The listing builds one solid part. Answer for the finished solid, in the listing's coordinates (mm). A direction names the side the tool comes from. Round coordinates to 2 decimals unless told otherwise and drop trailing zeros. Write each loop counter-clockwise with the first axis right and the second up, starting at its lowest first coordinate (ties: lowest second). Pieces come first, ordered by that corner, then holes. Notation, with made-up numbers: (32, 6.5) - (42, 6.5) arc R25 ccw to (42, 45.5) - close; hole circle Ø9 at (45.25, -29.5). An arc over 180 degrees is marked (long way). Answer in a Markdown table with one row per item.
from build123d import *

# Parameters (mm, degrees)
BOSS_EXTRUDE1_DEPTH  = 100
BOSS_EXTRUDE2_DEPTH  = 10
BOSS_EXTRUDE2_DRAFT  = 45
SKETCH3_R            = 34.5
BOSS_EXTRUDE3_DEPTH  = 10
SKETCH4_R            = 31
BOSS_EXTRUDE4_DEPTH  = 30
SKETCH5_R            = 2.5
SKETCH5_R_2          = 2
BOSS_EXTRUDE5_DEPTH  = 1
CIRPATTERN1_COUNT    = 12
BOSS_EXTRUDE6_DEPTH  = 100
SKETCH7_R            = 31
BOSS_EXTRUDE7_DEPTH  = 10
SKETCH8_R            = 30
BOSS_EXTRUDE8_DEPTH  = 1
SKETCH9_R            = 31
BOSS_EXTRUDE9_DEPTH  = 10
SKETCH10_R           = 42.5
BOSS_EXTRUDE10_DEPTH = 10.5
BOSS_EXTRUDE11_DEPTH = 35
BOSS_EXTRUDE12_DEPTH = 40
CUT_EXTRUDE1_DEPTH   = 40
SKETCH14_R           = 15
CUT_EXTRUDE2_DEPTH   = 20
SKETCH15_R           = 15
CUT_EXTRUDE3_DEPTH   = 20


with BuildPart() as part:
    # Sketch1 → Boss-Extrude1 (new body)
    with BuildSketch(Plane(origin=(0, 0, 0), x_dir=(0, 0, -1), z_dir=(1, 0, 0))):
        with BuildLine():
            Line((-37.5, 45), (37.5, 45))
            ThreePointArc((37.5, 45), (45.880962103, 0), (37.5, -45))
            Line((37.5, -45), (-37.5, -45))
            ThreePointArc((-37.5, -45), (-45.880962103, 0), (-37.5, 45))
        make_face()
    extrude(amount=BOSS_EXTRUDE1_DEPTH)


with BuildPart() as boss_extrude2_tool:
    # Sketch2 → Boss-Extrude2 (with draft: the straight prism first)
    with BuildSketch(Plane(origin=(100, 0, 0), x_dir=(0, 0, -1), z_dir=(1, 0, 0))):
        with BuildLine():
            Line((37.5, 45), (-37.5, 45))
            ThreePointArc((-37.5, 45), (-45.880962103, 0), (-37.5, -45))
            Line((-37.5, -45), (37.5, -45))
            ThreePointArc((37.5, -45), (45.880962103, 0), (37.5, 45))
        make_face()
    extrude(amount=BOSS_EXTRUDE2_DEPTH)
    # Boss-Extrude2: the draft: its side faces are tilted about the plane it starts from
    boss_extrude2_sides = [boss_extrude2_tool.faces().sort_by_distance(p)[0] for p in [
        (105, -45, 0),
        (105, 0, -45.880962103),
        (105, 45, 0),
        (105, 0, 45.880962103),
    ]]
    draft(boss_extrude2_sides, Plane(origin=(100, 0, 0), x_dir=(0, 0, -1), z_dir=(1, 0, 0)), BOSS_EXTRUDE2_DRAFT)


with BuildPart() as part_1:
    add(part.part)

    # Boss-Extrude2: add boss_extrude2_tool
    add(boss_extrude2_tool.part)

    # Sketch3 → Boss-Extrude3 (add)
    with BuildSketch(Plane(origin=(110, 0, 0), x_dir=(0, 0, -1), z_dir=(1, 0, 0))):
        Circle(SKETCH3_R)
    extrude(amount=BOSS_EXTRUDE3_DEPTH)

    # Sketch4 → Boss-Extrude4 (add)
    with BuildSketch(Plane(origin=(120, 0, 0), x_dir=(0, 0, -1), z_dir=(1, 0, 0))):
        Circle(SKETCH4_R)
    extrude(amount=BOSS_EXTRUDE4_DEPTH)

    # Sketch5 → Boss-Extrude5 (add)
    with BuildSketch(Plane(origin=(150, 0, 0), x_dir=(0, 0, -1), z_dir=(1, 0, 0))):
        with Locations((27, 0)):
            Circle(SKETCH5_R)
        with Locations((27, 0)):
            Circle(SKETCH5_R_2, mode=Mode.SUBTRACT)
    boss_extrude5 = extrude(amount=BOSS_EXTRUDE5_DEPTH)

    # CirPattern1: Boss-Extrude5 ×12 about axis
    cirpattern1_axis = Axis((0, 0, 0.17674784), (1, 0, 0))
    for i in range(1, CIRPATTERN1_COUNT):
        add(boss_extrude5.rotate(cirpattern1_axis, i * 360 / CIRPATTERN1_COUNT))

    # Sketch6 → Boss-Extrude6 (add)
    with BuildSketch(Plane(origin=(150, 0, 0), x_dir=(0, 0, -1), z_dir=(1, 0, 0))):
        with BuildLine():
            Line((16, 0), (16, 17))
            ThreePointArc((16, 17), (0, 23.900331129), (-16, 17))
            Line((-16, 17), (-16, 0))
            Line((-16, 0), (-16, -17))
            ThreePointArc((-16, -17), (0, -23.900331129), (16, -17))
            Line((16, -17), (16, 0))
        make_face()
    extrude(amount=BOSS_EXTRUDE6_DEPTH)

    # Sketch7 → Boss-Extrude7 (add)
    with BuildSketch(Plane(origin=(250, 0, 0), x_dir=(0, 0, -1), z_dir=(1, 0, 0))):
        Circle(SKETCH7_R)
    extrude(amount=BOSS_EXTRUDE7_DEPTH)

    # Sketch8 → Boss-Extrude8 (add)
    with BuildSketch(Plane(origin=(260, 0, 0), x_dir=(0, 0, -1), z_dir=(1, 0, 0))):
        Circle(SKETCH8_R)
    extrude(amount=BOSS_EXTRUDE8_DEPTH)

    # Sketch9 → Boss-Extrude9 (add)
    with BuildSketch(Plane(origin=(261, 0, 0), x_dir=(0, 0, -1), z_dir=(1, 0, 0))):
        Circle(SKETCH9_R)
    extrude(amount=BOSS_EXTRUDE9_DEPTH)

    # Sketch10 → Boss-Extrude10 (add, symmetric)
    with BuildSketch(Plane.XY.offset(37.5)):
        with Locations((50, -45)):
            Circle(SKETCH10_R)
    extrude(amount=BOSS_EXTRUDE10_DEPTH, both=True)

    # Sketch11 → Boss-Extrude11 (add)
    with BuildSketch(Plane(origin=(0, 0, 27), x_dir=(-1, 0, 0), z_dir=(0, 0, -1))):
        with BuildLine():
            Line((-62.06556146, -45), (-22.06556146, -45))
            Line((-22.06556146, -45), (-22.06556146, -75))
            ThreePointArc((-22.06556146, -75), (-42.06556146, -82.639320225), (-62.06556146, -75))
            Line((-62.06556146, -75), (-62.06556146, -45))
        make_face()
    extrude(amount=BOSS_EXTRUDE11_DEPTH)

    # Sketch12 → Boss-Extrude12 (add)
    with BuildSketch(Plane(origin=(62.06556146, 0, 0), x_dir=(0, 0, -1), z_dir=(1, 0, 0))):
        with BuildLine():
            Line((8, -45), (33, -45))
            ThreePointArc((33, -45), (25.421855105, -68.929675658), (8, -87))
            Line((8, -87), (8, -45))
        make_face()
    extrude(amount=-BOSS_EXTRUDE12_DEPTH)

    # Sketch13 → Cut-Extrude1 (cut)
    with BuildSketch(Plane.XY.offset(-8)):
        with BuildLine():
            Line((22.06556146, -75), (22.06556146, -87))
            Line((22.06556146, -87), (62.06556146, -87))
            Line((62.06556146, -87), (62.06556146, -75))
            ThreePointArc((62.06556146, -75), (42.06556146, -82.639320225), (22.06556146, -75))
        make_face()
    extrude(amount=-CUT_EXTRUDE1_DEPTH, mode=Mode.SUBTRACT)

    # Sketch14 → Cut-Extrude2 (cut)
    with BuildSketch(Plane(origin=(271, 0, 0), x_dir=(0, 0, -1), z_dir=(1, 0, 0))):
        Circle(SKETCH14_R)
    extrude(amount=-CUT_EXTRUDE2_DEPTH, mode=Mode.SUBTRACT)

    # Sketch15 → Cut-Extrude3 (cut)
    with BuildSketch(Plane.XY.offset(48)):
        with Locations((50, -45)):
            Circle(SKETCH15_R)
    extrude(amount=-CUT_EXTRUDE3_DEPTH, mode=Mode.SUBTRACT)


solid = part_1.part
(1) For faces 1 (the flat face through (68, -61, 27)), 2 (the flat face through (151, -12, 22)), 3 (the flat face through (251, 0, 0)), 4 (the flat face through (50, -45, 28)), 5 (the cylindrical face through (150.493, -21.095, -13.954)), determine the directions among +Z, -Z, +X, -X, +Y, -Y from which every point of the face is accessible in a straight line to the end or side of a thin tool.
Checked values:
| item | result |
|---|---|
| face 1 | -Z, -Y |
| face 2 | +Z, +Y, -Y |
| face 3 | +X |
| face 4 | +Z |
| face 5 | none |
(2) For a pull along X with two mould halves and no side action, classify faces 6 (the cylindrical face through (254.93, 30.736, 4.036)), 7 (the flat face through (62.066, -60, -3)), 8 (the cylindrical face through (150.49, -13.91, 26.19)) as pulls with the +X half, pulls with the -X half, needs draft (parallel to the pull), parting line crosses it, or undercut.
Checked values:
| item | result |
|---|---|
| face 6 | needs draft |
| face 7 | pulls with the +X half |
| face 8 | undercut |
(3) Flat-ended cylindrical pins translate along their axes: pin 1 (3 mm diameter, centred on x = 195, y = -18, fed in from -Z); pin 2 (12 mm diameter, centred on x = 43.5, y = -73.5, fed in from -Z); pin 3 (4 mm diameter, centred on x = 125.5, y = -23, fed in from +Z). Find the tip coordinate at first contact, or state that the pin passes through.
Checked values:
| item | result |
|---|---|
| pin 1 | stops at z = -16 |
| pin 2 | stops at z = -26.24 |
| pin 3 | stops at z = 22.8 |
(4) Section A-A (x = 45.5) is taken. Give the vertices of the cut face in (y, z).
Checked values:
| item | result |
|---|---|
| outline | (-87.26, 27) - (-82.44, 27) - (-82.44, -14.09) arc R55 ccw to (-45, -33) - (-45, -37.5) arc R125 ccw to (45, -37.5) - (45, 37.5) arc R125 ccw to (-2.74, 45.85) - (-2.74, 48) - (-30.69, 48) - (-30.69, 28) - (-59.31, 28) - (-59.31, 48) - (-87.26, 48) - close |
(5) Section B-B (y = -50.5) is taken. Give the vertices of the cut face in (x, z), and give its area (3 significant figures).
Checked values:
| item | result |
|---|---|
| outline | (7.86, 27) - (22.07, 27) - (22.07, -32.3) - (62.07, -32.3) - (62.07, 27) - (92.14, 27) - (92.14, 48) - (63.96, 48) - (63.96, 28) - (36.04, 28) - (36.04, 48) - (7.86, 48) - close |
| area | 3,580 mm2 |
(6) Section C-C (x = 209.5) is taken. Give the vertices of the cut face in (y, z).
Checked values:
| item | result |
|---|---|
| outline | (-17, -16) - (17, -16) arc R22 ccw to (17, 16) - (-17, 16) arc R22 ccw to start |
(7) Find the intervals of material crossed by line 1 (X direction, y = -17.5, z = -20.5); line 2 (X direction, y = 24, z = -29); line 3 (Y direction, x = 19, z = 16.5), in increasing order.
Checked values:
| item | result |
|---|---|
| line 1 | x = 0 to 150, 250 to 271 |
| line 2 | x = 0 to 110 |
| line 3 | y = -45 to 45 |
(8) Section D-D (y = -65) is taken. Give the vertices of the cut face in (x, z).
Checked values:
| item | result |
|---|---|
| outline | (12.5, 27) - (22.07, 27) - (22.07, -27.55) - (62.07, -27.55) - (62.07, 27) - (87.5, 27) - (87.5, 48) - (12.5, 48) - close |
